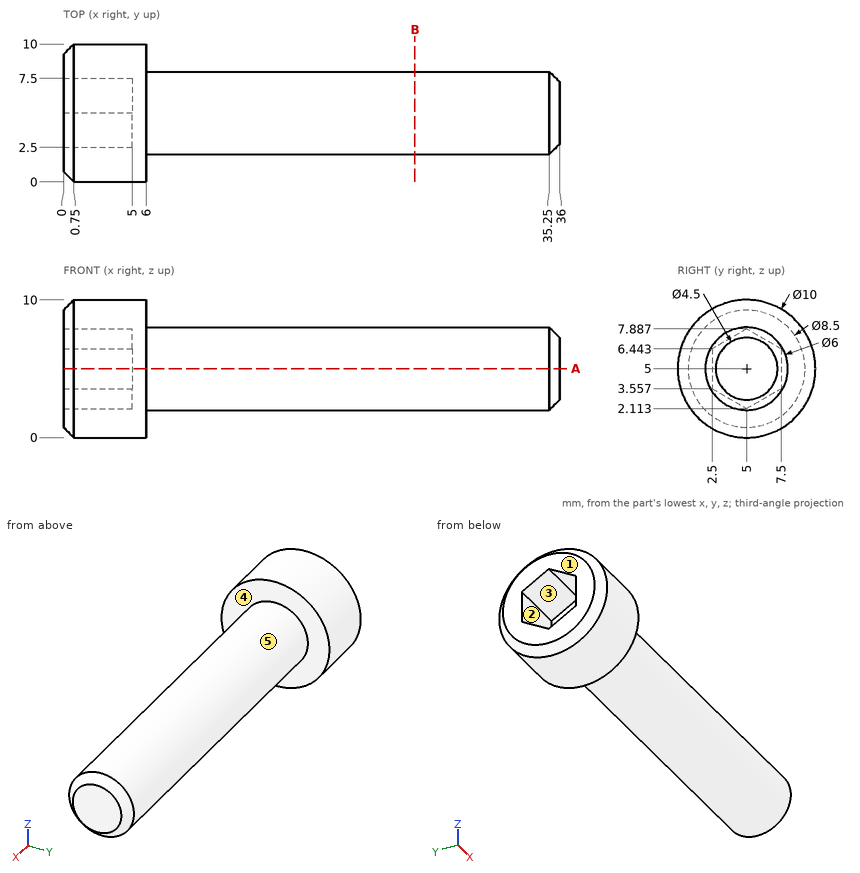
The figure shows three views and two pictorial views of one solid part (mm, origin at its lowest corner). Answer the questions. A direction names the side the tool comes from. Coordinates: 2 decimals unless noted, no trailing zeros. Loops run counter-clockwise (first coordinate to the right, second up) from the corner with the lowest first, then second, coordinate; pieces in that order, holes last.
(1) The part is cut by section A-A (z = 5). Determine the outline of the cut face in (x, y).
Solution:
outline: (0, 0.75) - (0.75, 0) - (6, 0) - (6, 2) - (35.25, 2) - (36, 2.75) - (36, 7.25) - (35.25, 8) - (6, 8) - (6, 10) - (0.75, 10) - (0, 9.25) - (0, 7.5) - (5, 7.5) - (5, 2.5) - (0, 2.5) - close
(2) The part is cut by section B-B (x = 25.5). Determine the outline of the cut face in (y, z), and give its area (3 significant figures).
Solution:
outline: circle Ø6 at (5, 5)
area: 28.3 mm2
(3) Flat-ended cylindrical pins translate along their axes: pin 1 Ø4 at (x, z) = (27, 3.5) entering from +Y; pin 2 Ø5 at (x, z) = (22, 4.5) entering from -Y; pin 3 Ø1.5 at (y, z) = (4.5, 4) entering from -X. Find the tip coordinate at first contact, or state that the pin passes through.
Solution:
pin 1: stops at y = 8
pin 2: stops at y = 2
pin 3: stops at x = 5
(4) A tool of negligible diameter and unlimited length cuts with its end or side. For the marked faces 1 and 2, from which of +Z, -Z, +X, -X, +Y, -Y can it reach the whole face along a straight path? Write none if from no direction.
Solution:
face 1: +Z, -Z, -X, +Y, -Y
face 2: -X
(5) Consider line 1 along X through (y, z) = (8.5, 4.25); line 2 along X through (y, z) = (3.25, 4.5); line 3 along Z through (x, y) = (33, 5). Determine where each line is inside the solid, lowest interval first.
Solution:
line 1: x = 0 to 6
line 2: x = 5 to 36
line 3: z = 2 to 8
(6) The mould has two halves that part along Z. Classify the marked faces 3, 4 and 5: released by +Z, released by -Z, zero draft, split by the parting line, or undercut.
Solution:
face 3: undercut
face 4: zero draft
face 5: split by the parting line
